```python
from build123d import *

# Parameters (mm, degrees)
SKETCH2_R           = 12.7
BOSS_EXTRUDE1_DEPTH = 38.1
SKETCH4_R           = 9.525
CUT_EXTRUDE1_DEPTH  = 19.05
SKETCH5_R           = 4.7625
CUT_EXTRUDE2_DEPTH  = 231.794329436
CHAMFER1_SIZE       = 0.254


with BuildPart() as part:
    # Sketch2 → Boss-Extrude1 (new body)
    with BuildSketch(Plane(origin=(0, 0, 0), x_dir=(1, 0, 0), z_dir=(0, 1, 0))):
        with BuildLine():
            Line((0, -25.4), (0, 25.4))
            Line((0, 25.4), (-101.6, 25.4))
            Line((-101.6, 25.4), (-101.6, 38.1))
            Line((-101.6, 38.1), (-76.2, 38.1))
            Line((-76.2, 38.1), (-0.116505732, 76.2))
            Line((-0.116505732, 76.2), (175.688681182, 76.2))
            ThreePointArc((175.688681182, 76.2), (187.352798222, 64.052185316), (196.85, 50.144482907))
            Line((196.85, 50.144482907), (196.85, 31.75))
            Line((196.85, 31.75), (171.986597881, 31.75))
            ThreePointArc((171.986597881, 31.75), (140.236597881, 0), (171.986597881, -31.75))
            Line((171.986597881, -31.75), (196.85, -31.75))
            Line((196.85, -31.75), (196.85, -50.144482907))
            ThreePointArc((196.85, -50.144482907), (187.352798222, -64.052185316), (175.688681182, -76.2))
            Line((175.688681182, -76.2), (-0.116505732, -76.2))
            Line((-0.116505732, -76.2), (-76.2, -38.1))
            Line((-76.2, -38.1), (-101.6, -38.1))
            Line((-101.6, -38.1), (-101.6, -25.4))
            Line((-101.6, -25.4), (0, -25.4))
        make_face()
        with Locations(Location((108.486597881, 0, 0), (0, 0, 90))):
            Circle(SKETCH2_R, mode=Mode.SUBTRACT)
    extrude(amount=BOSS_EXTRUDE1_DEPTH)

    # Sketch4 → Cut-Extrude1 (cut)
    with BuildSketch(Plane.ZY):
        with Locations((0, 19.05)):
            Circle(SKETCH4_R)
    extrude(amount=-CUT_EXTRUDE1_DEPTH, mode=Mode.SUBTRACT)

    # Sketch5 → Cut-Extrude2 (cut, through all)
    with BuildSketch(Plane.XY.offset(38.1)):
        with Locations((-88.9, 29.21)):
            Circle(SKETCH5_R)
        with Locations((-88.9, 8.89)):
            Circle(SKETCH5_R)
    extrude(amount=-CUT_EXTRUDE2_DEPTH, mode=Mode.SUBTRACT)

    # Chamfer1
    chamfer1_edges = [part.edges().sort_by_distance(p)[0] for p in [
        (108.486597881, 0, 12.7),
        (108.486597881, 38.1, 12.7),
        (0, 19.05, -9.525),
        (-93.6625, 29.21, -38.1),
        (-93.6625, 29.21, -25.4),
        (-93.6625, 29.21, 38.1),
        (-93.6625, 8.89, -38.1),
        (-93.6625, 8.89, -25.4),
        (-93.6625, 8.89, 25.4),
        (-93.6625, 8.89, 38.1),
    ]]
    chamfer(chamfer1_edges, length=CHAMFER1_SIZE)


solid = part.part
```
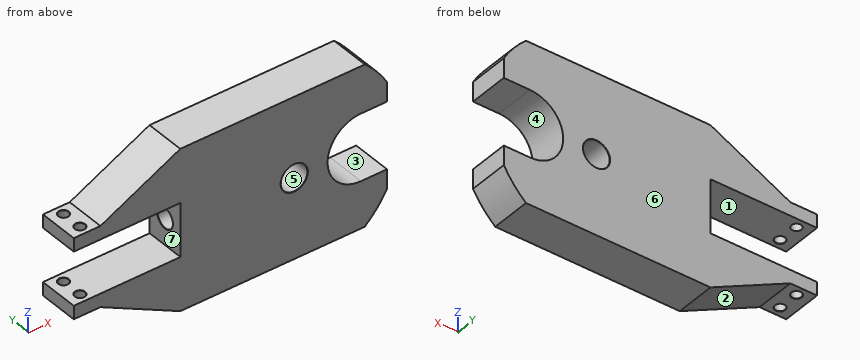
Part model, mm, in its own coordinate system. Face numbers are marked on the shaded views. A direction names the side the tool comes from. Give positions to 0.01 mm unless a question says otherwise; leave off trailing zeros. Write each loop counter-clockwise with the first axis right and the second up, starting at its lowest first coordinate (ties: lowest second). Pieces come first, ordered by that corner, then holes. Notation, with made-up numbers: (12, -37.75) -> (68, -37.75) arc R25 ccw to (68, -17.75) -> close; hole circle Ø8 at (24, 27.25). An arc over 180 degrees is marked (long way). Put each result on its own line as item: value. Start each with the question number.
Item 1: Cut at D-D (x = -88.9). State how many separate pieces and enclosed holes the cut face has, then the cut area to 3 significant figures.
Item 2: Wall check: L1, parallel to Y at x = -88.9, z = -33.5; L2, parallel to Z at x = -87.5, y = 21.5; L3, parallel to X at y = 30, z = 0. Give the ranges that are in metal, low to high. Write a range as [from, to].
Item 3: Cut at B-B (x = 160). List the corners of the cut face in (y, z), then the cut area to 3 significant figures.
Item 4: Which spindle directions (+Z, -Z, +X, -X, +Y, -Y) get a long thin tool onto all of the face, cutting with end or side? Do the marked faces 1, 2 and 3. Say none if no direction does.
Item 5: Pull direction X, two halves, no side cores. Call the marked faces 4, 5, 6 and 7: pulls with the +X half, pulls with the -X half, needs draft (parallel to the pull), parting line crosses it, or undercut.
Item 6: Pin check, flat tips, straight feed: pin 1 Ø8 at (y, z) = (4, -17.5) entering from -X; pin 2 Ø10 at (y, z) = (9.5, 52.5) entering from +X; pin 3 Ø8 at (y, z) = (14, 44.5) entering from -X; pin 4 Ø11 at (x, y) = (-88.9, 29.21) entering from +Z. Stop position of each tip, or through.
Item 7: Cut at A-A (z = 0). List the corners of the cut face in (x, y) (3 decimals).
Answer list:
1. separate pieces: 6
1. enclosed holes: 0
1. area: 483 mm2
2. L1: y = [0, 4.13], [13.65, 24.45], [33.97, 38.1]
2. L2: z = [-38.1, -25.4], [25.4, 38.1]
2. L3: x = [0, 95.79], [121.19, 140.24]
3. outline: (0, -76.2) -> (38.1, -76.2) -> (38.1, -29.4) -> (0, -29.4) -> close; (0, 29.4) -> (38.1, 29.4) -> (38.1, 76.2) -> (0, 76.2) -> close
3. area: 3,570 mm2
4. face 1: -X, +Y, -Y
4. face 2: -Z, -X, +Y, -Y
4. face 3: +X, +Y, -Y
5. face 4: pulls with the +X half
5. face 5: undercut
5. face 6: needs draft
5. face 7: pulls with the -X half
6. pin 1: stops at x = 0
6. pin 2: stops at x = 196.85
6. pin 3: stops at x = -71.41
6. pin 4: stops at z = 38.1
7. outline: (0, 0) -> (95.533, 0) -> (95.787, 0.254) -> (95.787, 37.846) -> (95.533, 38.1) -> (0, 38.1) -> (0, 28.829) -> (0.254, 28.575) -> (19.05, 28.575) -> (19.05, 9.525) -> (0.254, 9.525) -> (0, 9.271) -> close; (121.187, 0.254) -> (121.441, 0) -> (140.237, 0) -> (140.237, 38.1) -> (121.441, 38.1) -> (121.187, 37.846) -> close
